Design review of the part built by this model. Coordinates are the model's own, in mm. A direction names the side the tool comes from. Round coordinates to 2 decimals unless told otherwise and drop trailing zeros. Order: outer loops, then holes, each group sorted by start corner. A loop starts at its lowest first (then second) coordinate and runs counter-clockwise, first axis right, second up. Notation, with made-up numbers: M -31,38 L 20,38 A19 ccw 20,48 Z; hole C -24,26.5 d11. An arc over 180 degrees is marked long. Write each question's results on one line, items separated by ' | '. Start each with the question number.
Item 1: Take a section at B-B, the plane y = -366.25. Write out the cut boundary in (x, z), plus the area to 3 significant figures.
Item 2: Take a section at C-C, the plane z = -5.5. Write out the cut boundary in (x, y), plus the area to 4 significant figures.
Item 3: Clearance check with flat-ended pins moving along their axes: pin 1 (6 mm diameter, centred on y = -365.5, z = -7, fed in from +X); pin 2 (4 mm diameter, centred on y = -364, z = -1.5, fed in from -X); pin 3 (1 mm diameter, centred on x = -8.5, z = -8, fed in from -Y); pin 4 (4 mm diameter, centred on x = -12.5, z = -2.5, fed in from -Y). State where each tip first meets the part, or that it passes through.
Item 4: Machinability: for faces 4 (the flat face through (-9, -375.32, -8)), 5 (the cylindrical face through (-9.01, -356.82, -1.43)), 6 (the flat face through (-10, -367.4, -5.7)), which of the approach directions +Z, -Z, +X, -X, +Y, -Y give a long, thin tool a straight path to every point of the face, cutting with its end or side? Answer none if there is none.
Item 5: Wall thickness on line 1 (Y direction, x = -9.2, z = -7.5); line 2 (Y direction, x = -9, z = -7.75); line 3 (X direction, y = -368.5, z = -0.75): over which ranges is each line inside the solid? List them lowest first. Write a range as [from, to].
Item 6: The part is to be moulded in two halves that separate along Z. For faces 1 (the flat face through (-13, -377, -15)), 2 (the flat face through (-9, -374, -10.048)), 3 (the flat face through (-13, -377, 0)), say which applies: +Z half, -Z half, draft (parallel to the pull), parting line (faces both ways), or undercut.
Item 7: Take a section at A-A, the plane z = -7.5. Write out the cut boundary in (x, y), plus the area to 3 significant figures.
Item 8: Take a section at D-D, the plane x = -13.25. Write out the cut boundary in (y, z).
```python
from build123d import *

# Parameters (mm, degrees)
DODANIE_WYCI_GNI_CIE1_DEPTH = 15
SZKIC2_R                    = 2.5
WYTNIJ_WYCI_GNI_CIE2_DEPTH  = 15
SZKIC4_W                    = 5.095426068
SZKIC4_H                    = 2.09659
WYTNIJ_WYCI_GNI_CIE4_DEPTH  = 15
ZAOKR_GLENIE1_R             = 5


with BuildPart() as part:
    # Szkic1 → Dodanie-wyciągnięcie1 (new body)
    with BuildSketch(Plane.XY):
        with BuildLine():
            Line((-21.454955104, -379.577351541), (-23.824138202, -380.384479307))
            Line((-23.824138202, -380.384479307), (-23.175429976, -382.288649415))
            Line((-23.175429976, -382.288649415), (-9.642739559, -377.669332371))
            ThreePointArc((-9.642739559, -377.669332371), (-8.449909807, -376.75404191), (-7.997789918, -375.320100819))
            Line((-7.997789918, -375.320100819), (-8, -355.320100819))
            Line((-8, -355.320100819), (-10, -355.320100819))
            Line((-10, -355.320100819), (-10, -375.320100819))
            ThreePointArc((-10, -375.320100819), (-10.078304277, -375.588750623), (-10.288690869, -375.773254713))
            Line((-10.288690869, -375.773254713), (-21.454955104, -379.577351541))
        make_face()
    extrude(amount=-DODANIE_WYCI_GNI_CIE1_DEPTH)

    # Szkic2 → Wytnij-wyciągnięcie2 (cut)
    with BuildSketch(Plane.ZY.offset(10)):
        with Locations((-7.5, -364.820100819)):
            Circle(SZKIC2_R)
    extrude(amount=-WYTNIJ_WYCI_GNI_CIE2_DEPTH, mode=Mode.SUBTRACT)

    # Szkic4 → Wytnij-wyciągnięcie4 (cut)
    with BuildSketch(Plane.ZY.offset(10)):
        with Locations((-7.500510709, -374.271805819)):
            Rectangle(SZKIC4_W, SZKIC4_H)
    extrude(amount=-WYTNIJ_WYCI_GNI_CIE4_DEPTH, mode=Mode.SUBTRACT)

    # Zaokrąglenie1
    zaokr_glenie1_edges = [part.edges().sort_by_distance(p)[0] for p in [
        (-9, -355.320100819, 0),
        (-9, -355.320100819, -15),
    ]]
    fillet(zaokr_glenie1_edges, radius=ZAOKR_GLENIE1_R)


solid = part.part
```
Results list:
1) outline: M -10,-15 L -8,-15 L -8,-9.55 L -10,-9.55 Z; M -10,-5.45 L -8,-5.45 L -8,0 L -10,0 Z | area: 21.8 mm²
2) outline: M -23.82,-380.38 L -23.18,-382.29 L -9.64,-377.67 A2.5 ccw -8,-375.32 L -10,-375.32 A0.5 cw -10.29,-375.77 Z; M -10,-373.22 L -8,-373.22 L -8,-366.32 L -10,-366.32 Z; M -10,-363.32 L -8,-363.32 L -8,-355.32 L -10,-355.32 Z | area: 62.15 mm²
3) pin 1: x = -8 | pin 2: x = -10 | pin 3: y = -377.32 | pin 4: y = -379.33
4) face 4: +X, -X | face 5: +Z, +X, -X, +Y | face 6: +Z, -Z, -X, +Y
5) line 1: [-377.46, -375.32], [-373.22, -367.32], [-362.32, -355.32] | line 2: [-377.32, -375.32], [-373.22, -367.31], [-362.33, -355.32] | line 3: [-10, -8]
6) face 1: -Z half | face 2: undercut | face 3: +Z half
7) outline: M -23.82,-380.38 L -23.18,-382.29 L -9.64,-377.67 A2.5 ccw -8,-375.32 L -10,-375.32 A0.5 cw -10.29,-375.77 Z; M -10,-373.22 L -8,-373.22 L -8,-367.32 L -10,-367.32 Z; M -10,-362.32 L -8,-362.32 L -8,-355.32 L -10,-355.32 Z | area: 58.1 mm²
8) outline: M -378.9,-15 L -376.78,-15 L -376.78,0 L -378.9,0 Z
